Verification items for the finished model (mm, model axes). Coordinates: 2 decimals unless noted, no trailing zeros. Order: outer loops, then holes, each group sorted by start corner. A loop starts at its lowest first (then second) coordinate and runs counter-clockwise, first axis right, second up. Notation, with made-up numbers: M -17,-7 L -8,-7 A20 ccw -8,25 Z; hole C -15,-27 d1. An arc over 180 degrees is marked long. Return JSON: item names as keys, results as strings. Group by question number.
Q1. Thickness scan on probe 1 along Y at (x, z) = (-3.5, 1.2); probe 2 along X at (y, z) = (2, 2.7). Record the ranges inside material, lowest first.
Q2. Section check A-A, the plane z = 0. Enter the section's corners in (x, y), then the cut area to 3 significant figures.
Q3. Section check B-B, the plane x = 4. Enter the section's corners in (y, z).
Q4. Go/stop test with a flat-tipped pin: pin 1 Ø1.8 at (x, z) = (1.5, 0.5) entering from -Y. Record where the tip stops, or that it passes through.
Q5. Section check C-C, the plane z = 1.9. Enter the section's corners in (x, y).
Q6. Section check D-D, the plane x = -1. Enter the section's corners in (y, z).
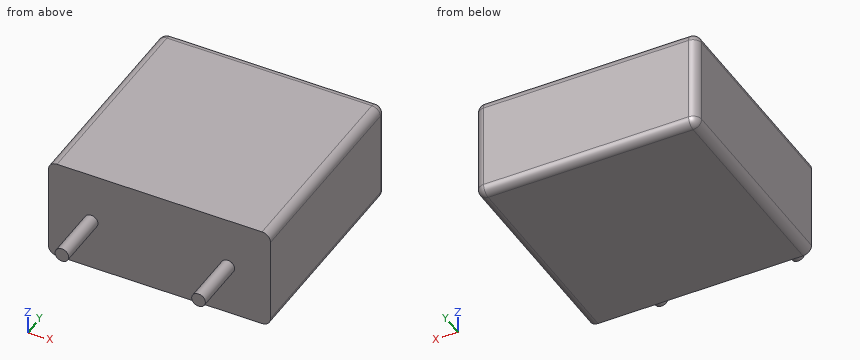
from build123d import *

# Parameters (mm, degrees)
SKETCH_2_W      = 13
SKETCH_2_H      = 6
EXTRUDE_1_DEPTH = 12.5
SKETCH_3_R      = 0.4
EXTRUDE_2_DEPTH = 3.2
FILLET_1_R      = 0.5


with BuildPart() as part:
    # Эскиз2 → Бобышка-Вытянуть1 (new body)
    with BuildSketch(Plane(origin=(0, 0, 0), x_dir=(1, 0, 0), z_dir=(0, 1, 0))):
        Rectangle(SKETCH_2_W, SKETCH_2_H)
    extrude(amount=EXTRUDE_1_DEPTH)

    # Эскиз3 → Бобышка-Вытянуть2 (add)
    with BuildSketch(Plane.XZ):
        with Locations(Location((-4, 0, 0), (0, 0, 270))):
            Circle(SKETCH_3_R)
        with Locations(Location((4, 0, 0), (0, 0, 270))):
            Circle(SKETCH_3_R)
    extrude(amount=EXTRUDE_2_DEPTH)

    # Скругление1
    fillet_1_edges = [part.edges().sort_by_distance(p)[0] for p in [
        (-6.5, 12.5, 0),
        (0, 12.5, 3),
        (6.5, 12.5, 0),
        (6.5, 6.25, 3),
        (-6.5, 6.25, 3),
        (-6.5, 6.25, -3),
        (6.5, 6.25, -3),
        (0, 12.5, -3),
    ]]
    fillet(fillet_1_edges, radius=FILLET_1_R)


solid = part.part
Numbers:
{
 "1": {"probe 1": "y = 0 to 12.5", "probe 2": "x = -6.46 to 6.46"},
 "2": {"outline": "M -6.5,0 L -4.4,0 L -4.4,-3.2 L -3.6,-3.2 L -3.6,0 L 3.6,0 L 3.6,-3.2 L 4.4,-3.2 L 4.4,0 L 6.5,0 L 6.5,12 A0.5 ccw 6,12.5 L -6,12.5 A0.5 ccw -6.5,12 Z", "area": "168 mm2"},
 "3": {"outline": "M -3.2,-0.4 L 0,-0.4 L 0,-3 L 12,-3 A0.5 ccw 12.5,-2.5 L 12.5,2.5 A0.5 ccw 12,3 L 0,3 L 0,0.4 L -3.2,0.4 Z"},
 "4": {"pin 1": "stops at y = 0"},
 "5": {"outline": "M -6.5,0 L 6.5,0 L 6.5,12 A0.5 ccw 6,12.5 L -6,12.5 A0.5 ccw -6.5,12 Z"},
 "6": {"outline": "M 0,-3 L 12,-3 A0.5 ccw 12.5,-2.5 L 12.5,2.5 A0.5 ccw 12,3 L 0,3 Z"}
}
